For this review, use the dimensioned drawing (mm, ordinates from the lowest corner) and the shaded views. A direction names the side the tool comes from. Coordinates: 2 decimals unless noted, no trailing zeros. Order: outer loops, then holes, each group sorted by start corner. A loop starts at its lowest first (then second) coordinate and runs counter-clockwise, first axis right, second up. Notation, with made-up numbers: M 60.5,65.5 L 72.5,65.5 A30 cw 72.5,103.5 Z; hole C 41,82 d4. An arc over 180 degrees is marked long. Answer in a Markdown table with one row per item.
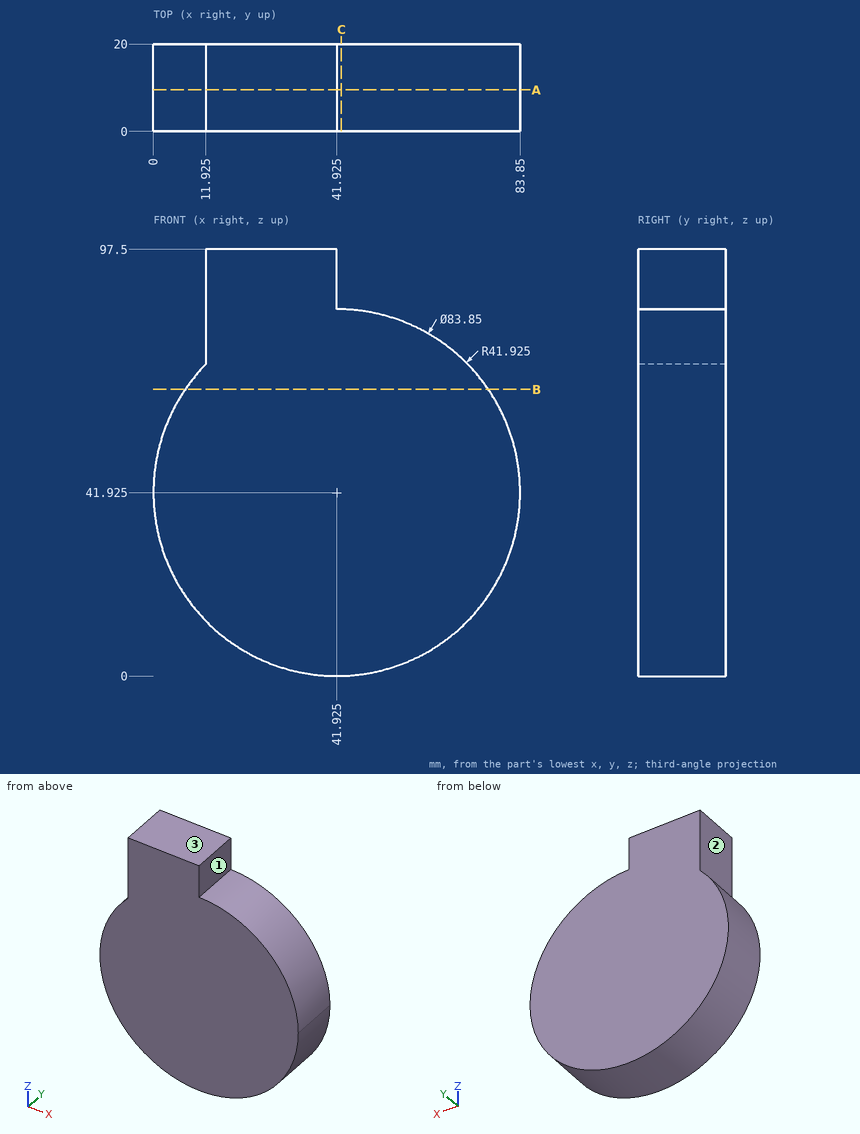
(1) Add section C-C, the plane x = 43. Give the boundary of the cut face in (y, z).
Return value:
| item | result |
|---|---|
| outline | M 0,0.01 L 20,0.01 L 20,83.84 L 0,83.84 Z |
(2) Insertion check: pin 1 Ø2 at (x, y) = (69, 16.5) entering from +Z; pin 2 Ø10 at (y, z) = (12, 87) entering from -X (3 decimals); pin 3 Ø5 at (y, z) = (15, 18) entering from -X. Each pin has a flat end and moves straight along its axis. Give the tip position at first contact, or say it passes through.
Return value:
| item | result |
|---|---|
| pin 1 | stops at z = 74.75 |
| pin 2 | stops at x = 11.925 |
| pin 3 | stops at x = 5.89 |
(3) For line 1 along Z through (x, y) = (10.5, 15.5); line 2 along X through (y, z) = (5.75, 9.5); line 3 along X through (y, z) = (3.25, 93.5) (3 decimals), list the stretches that pass through material, from the lowest coordinate up. Write a range as from..to.
Return value:
| item | result |
|---|---|
| line 1 | z = 14.17..69.68 |
| line 2 | x = 15.35..68.5 |
| line 3 | x = 11.925..41.925 |
(4) For the marked faces 1, 2 and 3, list the 3-axis set-ups (+Z, -Z, +X, -X, +Y, -Y) from which the entire face can be reached by the end or side of a thin tool; tool diameter is ignored.
Return value:
| item | result |
|---|---|
| face 1 | +Z, +X, +Y, -Y |
| face 2 | +Z, -X, +Y, -Y |
| face 3 | +Z, +X, -X, +Y, -Y |
(5) Add section A-A, the plane y = 9.5. Give the boundary of the cut face in (x, z) (3 decimals), and give its area (3 significant figures).
Return value:
| item | result |
|---|---|
| outline | M 11.925,71.212 A41.925 ccw long 41.925,83.85 L 41.925,97.5 L 11.925,97.5 Z |
| area | 6,050 mm2 |
(6) Add section B-B, the plane z = 65.5. Give the boundary of the cut face in (x, y), and give its area (3 significant figures).
Return value:
| item | result |
|---|---|
| outline | M 7.26,0 L 76.59,0 L 76.59,20 L 7.26,20 Z |
| area | 1,390 mm2 |
